For this review, take the finished solid that the model builds, in its own axes (mm). Give positions to 0.01 mm unless a question says otherwise; leave off trailing zeros. Use CSV: the item, a comma, the result in double quotes. Start each with the question number.
1. Mouldability with a two-part tool opening along Y and no side actions: class faces 1 (the cylindrical face through (120.753, 44.697, -1.232)), 2 (the flat face through (119, 53, -2.5)) as pulls with the +Y half, pulls with the -Y half, needs draft (parallel to the pull), parting line crosses it, or undercut.
2. Take a section at A-A on z = -1.7. State how many separate pieces and enclosed holes the cut face has, plus the area to 3 significant figures.
3. Wall thickness on line 1 (X direction, y = 40, z = -0.6); line 2 (Y direction, x = 209, z = -0.2); line 3 (Y direction, x = 162.5, z = -1.65): over which ranges is each line inside the solid? List them lowest first.
4. For pin 1 (1 mm diameter, centred on y = 44, z = -0.5, fed in from +X); pin 2 (4 mm diameter, centred on x = 238.9, y = 42.5, fed in from +Z); pin 3 (1.2 mm diameter, centred on y = 52, z = -1.5, fed in from +X), all flat-tipped, find the tip position at first contact; note any pin that passes through.
Autodesk Inventor part; units mm, degrees
ref_plane "YZ Plane" through (0, 0, 0) normal (1, 0, 0) x (0, 1, 0)
ref_plane "XZ Plane" through (0, 0, 0) normal (0, 1, 0) x (-1, 0, 0)
ref_plane "XY Plane" through (0, 0, 0) normal (0, 0, 1) x (1, 0, 0)
sketch "Skizze1" plane through (0, 0, 0) normal (0, 0, 1) x (1, 0, 0)
  line L0 (0, 0) -> (242, 0)
  line L1 (242, 0) -> (242, 85)
  line L2 (242, 85) -> (0, 85)
  line L3 (0, 85) -> (0, 0)
  line L4 (242, 42.5) -> (842, 42.5)
  line L5 (0, 42.5) -> (-937, 42.5)
  arc A0 (240, 0) -> (240, 85) centre (-210.5625, 42.5) ccw
  arc A1 (2, 85) -> (2, 0) centre (452.5625, 42.5) ccw
  dimension "d0" = 85
  dimension "d1" = 242
  dimension "d2" = 2
  dimension "d3" = 2
  dimension "d4" = 2
  dimension "d7" = 452.5625
  dimension "d8" = 452.5625
extrude "Extrusion1" add sketch "Skizze1" against normal blind 2.5 contours A1 L2 A0 L0
sketch "Skizze2" plane through (0, 0, 0) normal (0, 0, 1) x (1, 0, 0)
  line L0 (2, 0) -> (240, 0)
  line L1 (240, 85) -> (2, 85)
  line L2 (121, 0) -> (121, 85)
  point P0 (0, 0)
  point P1 (3.1, 42.5)
  point P2 (238.9, 42.5)
  dimension "d11" = 42.5
  dimension "d12" = 42.5
  dimension "d13" = 235.8
  dimension "d14" = 117.9
  dimension "d15" = 117.9
hole "Bohrung1" at (3.1, 42.5, 0) at (238.9, 42.5, 0) direction (0, 0, -1) diameter 3.3 depth 8 tip angle 118
sketch "Skizze3" plane through (0, 0, 0) normal (0, 0, 1) x (1, 0, 0)
  line L0 (2, 0) -> (240, 0)
  line L1 (240, 85) -> (2, 85)
  arc A0 (2, 85) -> (2, 0) centre (452.5625, 42.5) ccw
  line L2 (8.1386, 91.5936) -> (-1.2688, 78.1585)
  line L3 (-1.2688, 78.1585) -> (-1.2688, 91.5936)
  line L4 (-1.2688, 91.5936) -> (8.1386, 91.5936)
  line L5 (-1.7926, 7.5896) -> (9.0296, -7.8661)
  line L6 (9.0296, -7.8661) -> (-1.7926, -7.8661)
  line L7 (-1.7926, -7.8661) -> (-1.7926, 7.5896)
  line L8 (121, 0) -> (121, 85)
  line L9 (233.8614, 91.5936) -> (243.2688, 78.1585)
  line L10 (243.2688, 78.1585) -> (243.2688, 91.5936)
  line L11 (243.2688, 91.5936) -> (233.8614, 91.5936)
  line L12 (243.7926, 7.5896) -> (232.9704, -7.8661)
  line L13 (232.9704, -7.8661) -> (243.7926, -7.8661)
  line L14 (243.7926, -7.8661) -> (243.7926, 7.5896)
  point P0 (0, 0)
  point P1 (1.7712, 82.5)
  point P2 (1.7712, 2.5)
  point P3 (242, 0)
  point P4 (240.2288, 82.5)
  point P5 (240.2288, 2.5)
  dimension "d23" = 55
  dimension "d24" = 55
  dimension "d25" = 2.5
  dimension "d26" = 2.5
extrude "Extrusion2" cut sketch "Skizze3" against normal blind 5 contours A0 L5 L0 | L0 L5 L6 L7 A0 | L9 L11 L10 | L12 L14 L13 | L2 L3 L4 L1 A0 | A0 L1 L2
sketch "Sketch7" plane through (0, 0, 0) normal (0, 0, 1) x (1, 0, 0)
  point P0 (0, 0)
sketch "Sketch8" plane through (0, 0, 0) normal (0, 0, 1) x (1, 0, 0)
  circle A0 centre (151.8283, 22) radius 1.6
  line L0 (151.8283, 22) -> (227.3283, 22)
  circle A1 centre (227.3283, 22) radius 1.6
  line L1 (220.4783, 36.6) -> (158.6783, 36.6)
  line L2 (155.5783, 33.5) -> (155.5783, 10.5)
  line L3 (158.6783, 7.4) -> (220.4783, 7.4)
  line L4 (223.5783, 10.5) -> (223.5783, 33.5)
  line L5 (223.5783, 36.6) -> (155.5783, 7.4) construction
  line L6 (155.5783, 36.6) -> (223.5783, 7.4) construction
  arc A2 (158.6783, 36.6) -> (155.5783, 33.5) centre (158.6783, 33.5) ccw
  arc A3 (155.5783, 10.5) -> (158.6783, 7.4) centre (158.6783, 10.5) ccw
  arc A4 (220.4783, 7.4) -> (223.5783, 10.5) centre (220.4783, 10.5) ccw
  arc A5 (223.5783, 33.5) -> (220.4783, 36.6) centre (220.4783, 33.5) ccw
  line L7 (3.5217, 0) -> (238.4783, 0)
  line L8 (222.5783, 45) -> (177.5783, 45)
  line L9 (177.5783, 45) -> (177.5783, 61.5)
  line L10 (177.5783, 61.5) -> (222.5783, 61.5)
  line L11 (222.5783, 61.5) -> (222.5783, 45)
  line L12 (222.5783, 45) -> (177.5783, 61.5) construction
  line L13 (177.5783, 45) -> (222.5783, 61.5) construction
  line L14 (214.0783, 45) -> (186.0783, 45)
  line L15 (186.0783, 45) -> (186.0783, 61.5)
  line L16 (186.0783, 61.5) -> (214.0783, 61.5)
  line L17 (214.0783, 61.5) -> (214.0783, 45)
  line L18 (214.0783, 45) -> (186.0783, 61.5) construction
  line L19 (186.0783, 45) -> (214.0783, 61.5) construction
  circle A6 centre (217.5783, 55.5) radius 1.6
  circle A7 centre (182.5783, 55.5) radius 1.6
  arc A8 (122.7845, 17.85) -> (118.3721, 17.85) centre (120.5783, 22) ccw
  line L20 (118.3721, 17.85) -> (122.7845, 17.85)
  arc A9 (92.7845, 17.85) -> (88.3721, 17.85) centre (90.5783, 22) ccw
  line L21 (88.3721, 17.85) -> (92.7845, 17.85)
  arc A10 (107.7845, 17.85) -> (103.3721, 17.85) centre (105.5783, 22) ccw
  line L22 (103.3721, 17.85) -> (107.7845, 17.85)
  arc A11 (122.7845, 35.85) -> (118.3721, 35.85) centre (120.5783, 40) ccw
  line L23 (118.3721, 35.85) -> (122.7845, 35.85)
  line L24 (88.3721, 35.85) -> (92.7845, 35.85)
  arc A12 (92.7845, 35.85) -> (88.3721, 35.85) centre (90.5783, 40) ccw
  line L25 (103.3721, 35.85) -> (107.7845, 35.85)
  arc A13 (107.7845, 35.85) -> (103.3721, 35.85) centre (105.5783, 40) ccw
  point P0 (0, 0)
  point P1 (189.5783, 22)
  point P2 (200.0783, 53.25)
  dimension "d75" = 3.2
  dimension "d76" = 75.5
  dimension "d77" = 3.2
  dimension "d78" = 68
  dimension "d79" = 29.2
  dimension "d80" = 3.1
  dimension "d81" = 22
  dimension "d82" = 11.15
  dimension "d87" = 45
  dimension "d89" = 28
  dimension "d90" = 16.5
  dimension "d91" = 3.2
  dimension "d92" = 5
  dimension "d93" = 3.2
  dimension "d94" = 5
  dimension "d95" = 10.5
  dimension "d96" = 10.5
  dimension "d97" = 45
  dimension "d98" = 1
  dimension "d99" = 9.4
  dimension "d101" = 9.4
  dimension "d103" = 9.4
  dimension "d113" = 35
  dimension "d114" = 15
  dimension "d115" = 15
  dimension "d116" = 9.4
  dimension "d118" = 9.4
  dimension "d120" = 9.4
  dimension "d122" = 15
  dimension "d123" = 15
  dimension "d125" = 22
  dimension "d126" = 40
  dimension "d128" = 8.85
  dimension "d129" = 4.15
extrude "Extrusion5" cut sketch "Sketch8" against normal blind 3 contours A0 | A1 | L2 A2 L1 A5 L4 L0 | L0 L4 A4 L3 A3 L2 | L8 L15 L10 L17 | A6 | A7 | L20 A8 | L21 A9 | L22 A10 | L23 A11 | A12 L24 | A13 L25
properties part number "Frontplatte Apra Xdream 418"
Check result:
1,face 1,"undercut"
1,face 2,"needs draft"
2,separate pieces,"1"
2,enclosed holes,"14"
2,area,"17,600 mm²"
3,line 1,"x = 0.01 to 85.88, 95.28 to 100.88, 110.28 to 115.88, 125.28 to 241.99"
3,line 2,"y = 0 to 7.4, 36.6 to 45, 61.5 to 85"
3,line 3,"y = 0 to 7.4, 36.6 to 85"
4,pin 1,"stops at x = 242"
4,pin 2,"stops at z = 0"
4,pin 3,"stops at x = 241.91"
